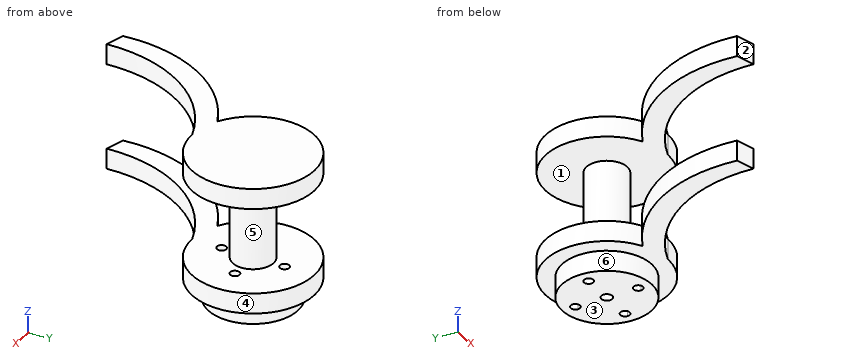
Autodesk Inventor part; units mm, degrees
ref_plane "YZ Plane" through (0, 0, 0) normal (1, 0, 0) x (0, 1, 0)
ref_plane "XZ Plane" through (0, 0, 0) normal (0, 1, 0) x (-1, 0, 0)
ref_plane "XY Plane" through (0, 0, 0) normal (0, 0, 1) x (1, 0, 0)
sketch "Esquisse1" plane through (0, 0, 0) normal (0, 0, 1) x (1, 0, 0)
  circle A0 centre (0, 0) radius 1.35
  circle A1 centre (0, -7.75) radius 1.15
  circle A2 centre (7.75, 0) radius 1.15
  circle A3 centre (0, 7.75) radius 1.15
  circle A4 centre (-7.75, 0) radius 1.15
  circle A5 centre (0, 0) radius 11
extrude "Extrusion1" add sketch "Esquisse1" along normal blind 10
sketch "Esquisse3" plane through (0, 0, 10) normal (0, 0, 1) x (1, 0, 0)
  circle A0 centre (0, 0) radius 1.35
  arc A1 (0, -15) -> (-7.3469, -13.0776) centre (0, 0) ccw
  arc A2 (-7.3469, -13.0776) -> (-27.8845, -48.1677) centre (6.8982, -44.9701) ccw
  arc A3 (0, -15) -> (-23.2475, -49.4967) centre (11.2565, -47.6674) ccw
  line L0 (-27.8845, -48.1677) -> (-23.2475, -49.4967)
  dimension "d28" = 30
extrude "Extrusion3" add sketch "Esquisse3" along normal blind 5
sketch "Esquisse4" plane through (0, 0, 0) normal (0, 0, -1) x (-1, 0, 0)
  circle A0 centre (0, 0) radius 1.35
  circle A1 centre (7.75, 0) radius 1.15
  circle A2 centre (0, 7.75) radius 1.15
  circle A3 centre (-7.75, 0) radius 1.15
  circle A4 centre (0, -7.75) radius 1.15
  circle A5 centre (0, 0) radius 11
extrude "Extrusion4" cut sketch "Esquisse4" against normal blind 46.25 contours A0 | A1 | A2 | A3 | A4
sketch "Esquisse5" plane through (0, 0, 15) normal (0, 0, 1) x (1, 0, 0)
  circle A0 centre (0, 0) radius 5
  dimension "d33" = 10
extrude "Extrusion5" add sketch "Esquisse5" along normal blind 26
pattern_linear "Réseau rectangulaire1" count 2 spacing 26 along (0, 0, 1) of "Extrusion3"
sketch "Esquisse6" plane through (0, 0, 0) normal (0, 0, -1) x (-1, 0, 0)
  circle A0 centre (0, 0) radius 1.35
  circle A1 centre (0, 0) radius 11
extrude "Extrusion6" cut sketch "Esquisse6" against normal blind 5
properties part number "carroussel"
The model under review builds one solid part; all positions refer to its coordinate system, in mm. Face numbers are marked on the shaded views. A direction names the side the tool comes from. Coordinates: 2 decimals unless noted, no trailing zeros. Write each loop counter-clockwise with the first axis right and the second up, starting at its lowest first coordinate (ties: lowest second). Pieces come first, ordered by that corner, then holes.
1) We need section C-C on z = 23. State the section outline as (x, y) points, then the cut area to 3 significant figures.
2) Clearance check with flat-ended pins moving along their axes: pin 1 Ø1.8 at (x, y) = (0, -7.75) entering from -Z; pin 2 Ø1.6 at (x, y) = (0, 0) entering from -Z; pin 3 Ø5 at (x, z) = (2.5, 22.5) entering from -Y. State where each tip first meets the part, or that it passes through.
3) We need section B-B on x = -10. State the section outline as (y, z) points.
4) The part is to be moulded in two halves that separate along Z. For the marked faces 1, 2 and 3, say which applies: pulls with the +Z half, pulls with the -Z half, needs draft (parallel to the pull), parting line crosses it, or undercut.
5) Machinability: for the marked faces 4, 5 and 6, which of the approach directions +Z, -Z, +X, -X, +Y, -Y give a long, thin tool a straight path to every point of the face, cutting with its end or side? Answer none if there is none.
6) We need section D-D on x = 4. State the section outline as (y, z) points.
7) We need section A-A on x = -18. State the section outline as (y, z) points, then the cut area to 3 significant figures.
8) To check wall thickness, follow probe 1 along X at (y, z) = (0, 13); probe 2 along Z at (x, y) = (-12.5, 4). State the ranges of each line that lie inside material, in increasing order.
Answer list:
1. outline: circle Ø10 at (0, 0)
1. area: 78.5 mm2
2. pin 1: stops at z = 36
2. pin 2: stops at z = 15
2. pin 3: stops at y = -5
3. outline: (-20.43, 10) - (-14.4, 10) - (-14.4, 15) - (-20.43, 15) - close; (-20.43, 36) - (-14.4, 36) - (-14.4, 41) - (-20.43, 41) - close; (-11.18, 10) - (-4.58, 10) - (-4.58, 5) - (4.58, 5) - (4.58, 10) - (11.18, 10) - (11.18, 15) - (-11.18, 15) - close; (-11.18, 36) - (11.18, 36) - (11.18, 41) - (-11.18, 41) - close
4. face 1: undercut
4. face 2: needs draft
4. face 3: pulls with the -Z half
5. face 4: +Z, -Z
5. face 5: none
5. face 6: -Z
6. outline: (-14.46, 10) - (-10.25, 10) - (-10.25, 5) - (10.25, 5) - (10.25, 10) - (14.46, 10) - (14.46, 15) - (3, 15) - (3, 36) - (14.46, 36) - (14.46, 41) - (-14.46, 41) - (-14.46, 36) - (-3, 36) - (-3, 15) - (-14.46, 15) - close
7. outline: (-29.28, 10) - (-20.47, 10) - (-20.47, 15) - (-29.28, 15) - close; (-29.28, 36) - (-20.47, 36) - (-20.47, 41) - (-29.28, 41) - close
7. area: 88.1 mm2
8. probe 1: x = -15 to -8.9, -6.6 to -1.35, 1.35 to 6.6, 8.9 to 15
8. probe 2: z = 10 to 15, 36 to 41
